Geometry check sheet. Reference: drawing and pictorial views, mm from the part's lowest x, y, z. A direction names the side the tool comes from. Give positions to 0.01 mm unless a question says otherwise; leave off trailing zeros. Write each loop counter-clockwise with the first axis right and the second up, starting at its lowest first coordinate (ties: lowest second). Pieces come first, ordered by that corner, then holes. Notation, with made-up numbers: M 65,-17.5 L 116,-17.5 A14 cw 116,4.5 Z; hole C -30.5,-0.75 d9. An arc over 180 degrees is marked long. Write item = value, one per line. Start each with the question number.
1) Cross-section at B-B, the plane x = 4.25. Record the cut outline in (y, z), plus the area to 3 significant figures.
2) Go/stop test with flat-tipped pins: pin 1 (1.5 mm diameter, centred on x = 8, z = 4, fed in from -Y); pin 2 (1.5 mm diameter, centred on x = 5.5, z = 7, fed in from +Y); pin 3 (5 mm diameter, centred on x = 8, y = 6.5, fed in from -Z). Record where each tip stops, or that it passes through.
3) Scan lines: line 1 along X through (y, z) = (7.75, 3.5); line 2 along Z through (x, y) = (7.75, 5.75); line 3 along Y through (x, z) = (6, 1.75) (1 decimal). Record each from-to range of solid material in increasing order. Write a range as [from, to].
4) Cross-section at A-A, the plane x = 2. Record the cut outline in (y, z).
5) Access from +Z, -Z, +X, -X, +Y, -Y to the whole of each face (thin tool, end or side, straight path). Record for the marked faces 1 and 2.
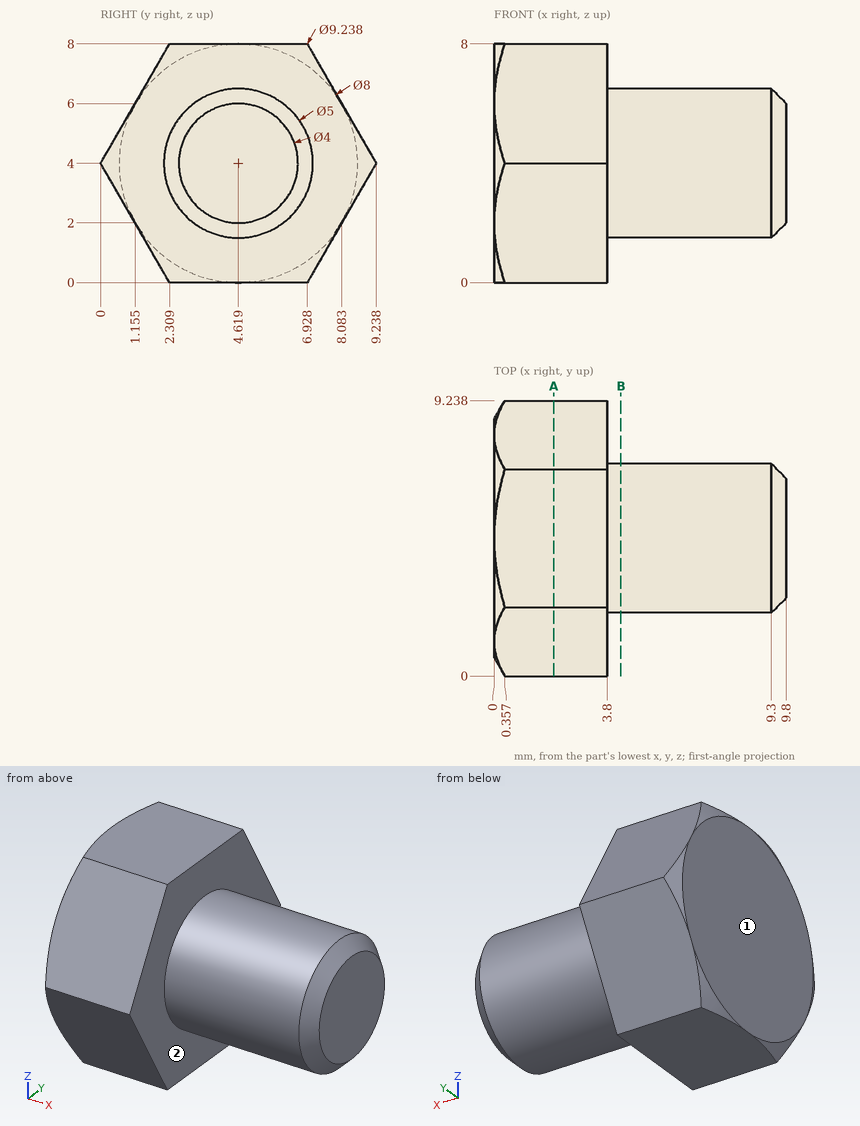
Reply:
q1.outline = C 4.62,4 d5
q1.area = 19.6 mm2
q2.pin_1 = 2.12
q2.pin_2 = 5.71
q2.pin_3 = 1.5
q3.line_1 = [0, 3.8]
q3.line_2 = [1.77, 6.23]
q3.line_3 = [3.5, 5.7]
q4.outline = M 0,4 L 2.31,0 L 6.93,0 L 9.24,4 L 6.93,8 L 2.31,8 Z
q5.face_1 = +Z, -Z, -X, +Y, -Y
q5.face_2 = +X
